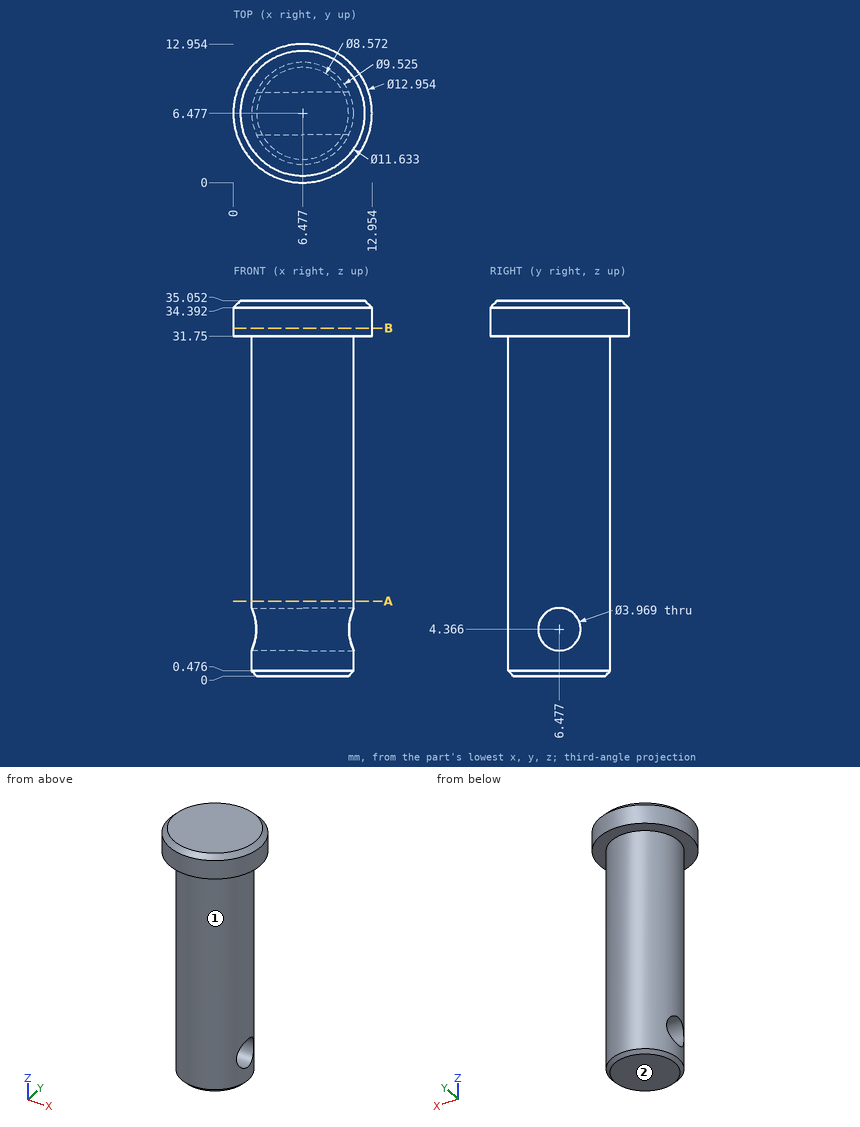
Study the drawing (mm; zero at the part's minimum x, y, z) and answer. A direction names the side the tool comes from. Round coordinates to 2 decimals unless told otherwise and drop trailing zeros. Loops run counter-clockwise (first coordinate to the right, second up) from the corner with the lowest first, then second, coordinate; pieces in that order, holes last. Notation, with made-up numbers: M -38,61.25 L -1,61.25 A25 cw -1,74.25 Z; hole C 3,-2.75 d6. An arc over 180 degrees is marked long. One line per question, with ' | ' between items.
Q1. Consider line 1 along Z through (x, y) = (5.25, 5.5); line 2 along Z through (x, y) = (5.5, 1.5); line 3 along X through (y, z) = (6.5, 28) (1 decimal). Determine where each line is inside the solid, lowest interval first. Write a range as from..to.
Conclusion:
line 1: z = 0..2.64, 6.09..35.05 | line 2: z = 31.75..35.05 | line 3: x = 1.7..11.2
Q2. Find section B-B, the plane z = 32.5. Give the vertices of the cut face in (x, y) (1 decimal), then the cut area to 3 significant figures.
Conclusion:
outline: C 6.5,6.5 d13 | area: 132 mm2
Q3. Each of these flat-tipped pins is pushed along its axis until it touches: pin 1 Ø6 at (x, y) = (4, 3) entering from -Z; pin 2 Ø2.5 at (y, z) = (6.48, 4.37) entering from -X; pin 3 Ø5 at (y, z) = (11.5, 18.5) entering from -X; pin 4 Ø1.5 at (y, z) = (8, 12.5) entering from -X. Where does it stop, or does it pass through?
Conclusion:
pin 1: stops at z = 0 | pin 2: passes through | pin 3: stops at x = 2.44 | pin 4: stops at x = 1.78
Q4. A tool of negligible diameter and unlimited length cuts with its end or side. For the marked faces 1 and 2, from which of +Z, -Z, +X, -X, +Y, -Y can it reach the whole face along a straight path? Write none if from no direction.
Conclusion:
face 1: -Z | face 2: -Z, +X, -X, +Y, -Y
Q5. Find section A-A, the plane z = 7. Give the vertices of the cut face in (x, y) (1 decimal).
Conclusion:
outline: C 6.5,6.5 d9.5
